```python
from build123d import *

# Parameters (mm, degrees)
F0_W     = 65
F0_H     = 128
F0_R     = 8
F1_DEPTH = 12
F2_R     = 16
F3_R     = 30
F3_R_2   = 26
F4_DEPTH = 46


with BuildPart() as f1:
    # F0 (on Top) → F1 (new body)
    with BuildSketch(Plane.XY):
        with Locations((-2.270288, 12.264718)):
            Rectangle(F0_W, F0_H)
        with Locations((-19.155467, -33.992235)):
            Circle(F0_R, mode=Mode.SUBTRACT)
        with Locations((13.844533, -33.992235)):
            Circle(F0_R, mode=Mode.SUBTRACT)
        with Locations((-19.155467, 62.007765)):
            Circle(F0_R, mode=Mode.SUBTRACT)
        with Locations((13.844533, 62.007765)):
            Circle(F0_R, mode=Mode.SUBTRACT)
    extrude(amount=F1_DEPTH)

    # F2
    f2_edges = [f1.edges().sort_by_distance(p)[0] for p in [
        (30.229712, -51.735282, 6),
        (-34.770288, -51.735282, 6),
        (-34.770288, 76.264718, 6),
        (30.229712, 76.264718, 6),
    ]]
    fillet(f2_edges, radius=F2_R)

    # F3 (on Top) → F4 (join)
    with BuildSketch(Plane.XY):
        with Locations((-2.270288, 12.264718)):
            Circle(F3_R)
        with Locations((-2.270288, 12.264718)):
            Circle(F3_R_2, mode=Mode.SUBTRACT)
    extrude(amount=F4_DEPTH)


solid = f1.part
```
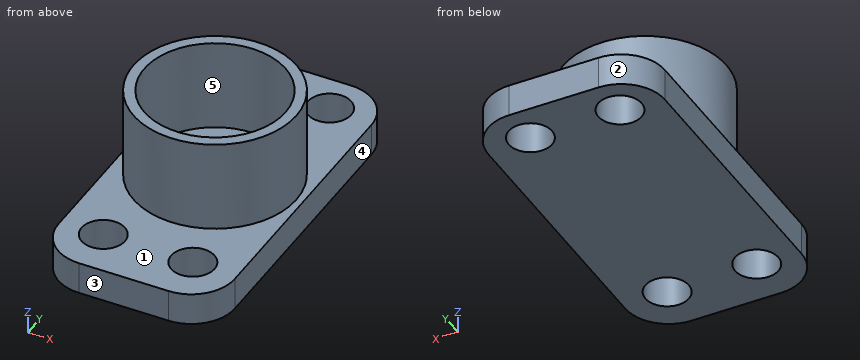
Check sheet for the modelled part. Datum: model origin and axes. Units: mm. Face numbers are marked on the shaded views. A direction names the side the tool comes from. Round coordinates to 2 decimals unless told otherwise and drop trailing zeros. Loops run counter-clockwise (first coordinate to the right, second up) from the corner with the lowest first, then second, coordinate; pieces in that order, holes last. Notation, with made-up numbers: (-26, -13.75) -> (30, -13.75) arc R26 ccw to (30, 10.25) -> close; hole circle Ø10 at (51.25, 40). An arc over 180 degrees is marked (long way). Answer in a Markdown table with one row per item.
Q1. Set-up check for the marked faces 1 and 2: record each of +Z, -Z, +X, -X, +Y, -Y from which the full face is reachable in a straight line by a thin tool's end or side.
Data:
| item | result |
|---|---|
| face 1 | +Z |
| face 2 | +Z, -Z, -X, +Y |
Q2. Go/stop test with flat-tipped pins: P1, Ø6, axis at x = 18, y = 56, coming from the +Z side; P2, Ø9.5, axis at x = -19.16, y = 62.01, coming from the -Z side; P3, Ø5, axis at y = 15.5, z = 32, coming from the +X side; P4, Ø1, axis at y = 19, z = 28, coming from the +X side. Record where each tip stops, or that it passes through.
Data:
| item | result |
|---|---|
| P1 | stops at z = 12 |
| P2 | passes through |
| P3 | stops at x = 27.72 |
| P4 | stops at x = 27.07 |
Q3. Thickness scan on L1, parallel to X at y = 12, z = 34; L2, parallel to Z at x = 21, y = 7.5; L3, parallel to Y at x = -14.5, z = 5.5. Record the ranges inside material, lowest first.
Data:
| item | result |
|---|---|
| L1 | x = -32.27 to -28.27, 23.73 to 27.73 |
| L2 | z = 0 to 12 |
| L3 | y = -51.74 to -40.5, -27.49 to 55.5, 68.51 to 76.26 |
Q4. Sectioned sample at C-C on y = 27.5. Enter the section's corners in (x, z).
Data:
| item | result |
|---|---|
| outline | (-34.77, 0) -> (30.23, 0) -> (30.23, 12) -> (23.57, 12) -> (23.57, 46) -> (18.8, 46) -> (18.8, 12) -> (-23.34, 12) -> (-23.34, 46) -> (-28.11, 46) -> (-28.11, 12) -> (-34.77, 12) -> close |
Q5. Sectioned sample at A-A on y = 66. Enter the section's corners in (x, z).
Data:
| item | result |
|---|---|
| outline | (-33.71, 0) -> (-26.09, 0) -> (-26.09, 12) -> (-33.71, 12) -> close; (-12.22, 0) -> (6.91, 0) -> (6.91, 12) -> (-12.22, 12) -> close; (20.78, 0) -> (29.17, 0) -> (29.17, 12) -> (20.78, 12) -> close |
Q6. Release check for a two-part mould opening along Y. For the marked faces 3, 4 and 5 record: released by +Y, released by -Y, zero draft, split by the parting line, or undercut.
Data:
| item | result |
|---|---|
| face 3 | released by -Y |
| face 4 | zero draft |
| face 5 | undercut |
Q7. Sectioned sample at D-D on x = -9. Enter the section's corners in (y, z).
Data:
| item | result |
|---|---|
| outline | (-51.74, 0) -> (76.26, 0) -> (76.26, 12) -> (41.5, 12) -> (41.5, 46) -> (37.38, 46) -> (37.38, 12) -> (-12.85, 12) -> (-12.85, 46) -> (-16.97, 46) -> (-16.97, 12) -> (-51.74, 12) -> close |
Q8. Sectioned sample at B-B on x = 15.5. Enter the section's corners in (y, z).
Data:
| item | result |
|---|---|
| outline | (-51.68, 0) -> (-41.82, 0) -> (-41.82, 12) -> (-51.68, 12) -> close; (-26.17, 0) -> (54.18, 0) -> (54.18, 12) -> (36.44, 12) -> (36.44, 46) -> (31.24, 46) -> (31.24, 12) -> (-6.71, 12) -> (-6.71, 46) -> (-11.91, 46) -> (-11.91, 12) -> (-26.17, 12) -> close; (69.83, 0) -> (76.21, 0) -> (76.21, 12) -> (69.83, 12) -> close |
